from build123d import *

# Parameters (mm, degrees)
SKETCH1_W           = 78
SKETCH1_H           = 88.5
SKETCH1_W_2         = 72
SKETCH1_H_2         = 82.5
BOSS_EXTRUDE1_DEPTH = 5
SKETCH2_W           = 78
SKETCH2_H           = 88.5
SKETCH2_R           = 1.6
SKETCH2_R_2         = 1.738
BOSS_EXTRUDE2_DEPTH = 2
SKETCH7_W           = 7.279998142
SKETCH7_H           = 50.36
SKETCH7_W_2         = 7.079999996
SKETCH7_H_2         = 50.160000192
CUT_EXTRUDE1_DEPTH  = 15
SKETCH9_W           = 7.45
SKETCH9_H           = 4.497118046
CUT_EXTRUDE7_DEPTH  = 16
SKETCH10_R          = 2.1
SKETCH10_R_2        = 2.238
BOSS_EXTRUDE4_DEPTH = 1
CUT_EXTRUDE8_START  = -15
SKETCH11_R          = 1.738
SKETCH11_R_2        = 1.6
CUT_EXTRUDE8_DEPTH  = 15


with BuildPart() as part:
    # Sketch1 → Boss-Extrude1 (new body)
    with BuildSketch(Plane.XY):
        with Locations((19.784172662, -18.690647482)):
            Rectangle(SKETCH1_W, SKETCH1_H)
        with Locations((19.784172662, -18.690647482)):
            Rectangle(SKETCH1_W_2, SKETCH1_H_2, mode=Mode.SUBTRACT)
    extrude(amount=BOSS_EXTRUDE1_DEPTH)

    # Sketch2 → Boss-Extrude2 (add)
    with BuildSketch(Plane(origin=(0, 0, 0), x_dir=(-1, 0, 0), z_dir=(0, 0, -1))):
        with Locations((-19.784172662, -18.690647482)):
            Rectangle(SKETCH2_W, SKETCH2_H)
        with Locations((4.233803916, -5.370645303)):
            Circle(SKETCH2_R, mode=Mode.SUBTRACT)
        with Locations((-44.026196036, -6.640647161)):
            Circle(SKETCH2_R_2, mode=Mode.SUBTRACT)
        with Locations((-28.78619408, -57.440646574)):
            Circle(SKETCH2_R_2, mode=Mode.SUBTRACT)
    extrude(amount=BOSS_EXTRUDE2_DEPTH)

    # Sketch7 → Cut-Extrude1 (cut)
    with BuildSketch(Plane.XY):
        with Locations((-10.583804942, -31.990645157)):
            Rectangle(SKETCH7_W, SKETCH7_H)
        with Locations((50.276195985, -32.090647407)):
            Rectangle(SKETCH7_W_2, SKETCH7_H_2)
    extrude(amount=-CUT_EXTRUDE1_DEPTH, mode=Mode.SUBTRACT)

    # Sketch9 → Cut-Extrude7 (cut)
    with BuildSketch(Plane.XZ.offset(-22.559352518)):
        with Locations((31.833296536, 2.751440977)):
            Rectangle(SKETCH9_W, SKETCH9_H)
    extrude(amount=-CUT_EXTRUDE7_DEPTH, mode=Mode.SUBTRACT)

    # Sketch10 → Boss-Extrude4 (add)
    with BuildSketch(Plane.XY):
        with Locations(Location((-4.233803916, -5.370645303, 0), (0, 0, 180))):
            Circle(SKETCH10_R)
        with Locations(Location((44.026196036, -6.640647161, 0), (0, 0, 180))):
            Circle(SKETCH10_R_2)
        with Locations(Location((28.78619408, -57.440646574, 0), (0, 0, 180))):
            Circle(SKETCH10_R_2)
    extrude(amount=BOSS_EXTRUDE4_DEPTH)

    # Sketch11 → Cut-Extrude8 (cut)
    with BuildSketch(Plane(origin=(0, 0, 0), x_dir=(-1, 0, 0), z_dir=(0, 0, -1)).offset(CUT_EXTRUDE8_START)):
        with Locations(Location((-44.026196036, -6.640647161, 0), (0, 0, 180))):
            Circle(SKETCH11_R)
        with Locations(Location((4.233803916, -5.370645303, 0), (0, 0, 180))):
            Circle(SKETCH11_R_2)
        with Locations(Location((-28.78619408, -57.440646574, 0), (0, 0, 180))):
            Circle(SKETCH11_R)
    extrude(amount=CUT_EXTRUDE8_DEPTH, mode=Mode.SUBTRACT)


solid = part.part
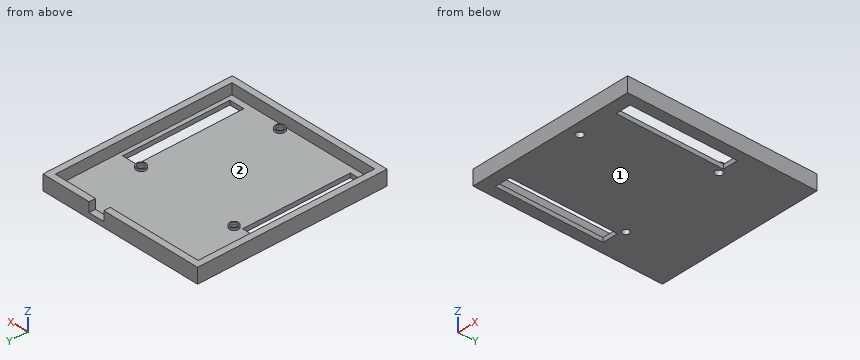
Model file for the job. Use its own axes, mm. Face numbers are marked on the shaded views. Give positions to 0.01 mm unless a question says otherwise; leave off trailing zeros. Order: outer loops, then holes, each group sorted by start corner. A loop starts at its lowest first (then second) coordinate and runs counter-clockwise, first axis right, second up. Notation, with made-up numbers: (29, 61.25) - (69, 61.25) arc R10 cw to (69, 75.25) - close; hole circle Ø8 at (-21.5, -24). An arc over 180 degrees is marked (long way). Return JSON: item names as keys, results as strings.
1) Cut at C-C, the plane z = 2.5. Give the cut face in (x, y).
Geometry says:
{"outline": "(-19.22, -62.94) - (58.78, -62.94) - (58.78, 25.56) - (35.56, 25.56) - (35.56, 22.56) - (55.78, 22.56) - (55.78, -59.94) - (-16.22, -59.94) - (-16.22, 22.56) - (28.11, 22.56) - (28.11, 25.56) - (-19.22, 25.56) - close"}
2) Flat gauge pins, fed straight in: P1, Ø3.5, axis at x = 45, y = -5.5, coming from the +Z side; P2, Ø8, axis at x = -1, y = -29, coming from the +Z side; P3, Ø1.5, axis at x = 32, y = 23.5, coming from the +Z side. Where does each tip first touch, or does it go through?
Geometry says:
{"P1": "z = 1", "P2": "z = 0", "P3": "z = 0.5"}
3) Probe line 1 (X direction, y = -10, z = -0.25); line 2 (Y direction, x = 2, z = 3.75); line 3 (X direction, y = -36, z = 4.25). List the from-to ranges inside material, lowest first. Write a range as from..to.
Geometry says:
{"line 1": "-19.22..-14.22, -6.94..46.74, 53.82..58.78", "line 2": "-62.94..-59.94, 22.56..25.56", "line 3": "-19.22..-16.22, 55.78..58.78"}
4) Cut at B-B, the plane y = -25. Give the cut face in (x, z).
Geometry says:
{"outline": "(-19.22, -2) - (-14.22, -2) - (-14.22, 0) - (-16.22, 0) - (-16.22, 5) - (-19.22, 5) - close; (-6.94, -2) - (46.74, -2) - (46.74, 0) - (-6.94, 0) - close; (53.82, -2) - (58.78, -2) - (58.78, 5) - (55.78, 5) - (55.78, 0) - (53.82, 0) - close"}
5) Pull direction X, two halves, no side cores. Call the marked faces 1 and 2: pulls with the +X half, pulls with the -X half, needs draft (parallel to the pull), parting line crosses it, or undercut.
Geometry says:
{"face 1": "needs draft", "face 2": "undercut"}
6) Cut at A-A, the plane x = 34. Give the cut face in (y, z).
Geometry says:
{"outline": "(-62.94, -2) - (25.56, -2) - (25.56, 0.5) - (22.56, 0.5) - (22.56, 0) - (-59.94, 0) - (-59.94, 5) - (-62.94, 5) - close"}
7) Cut at D-D, the plane y = 16.5. Give the cut face in (x, z), plus the area to 3 significant figures.
Geometry says:
{"outline": "(-19.22, -2) - (58.78, -2) - (58.78, 5) - (55.78, 5) - (55.78, 0) - (-16.22, 0) - (-16.22, 5) - (-19.22, 5) - close", "area": "186 mm²"}
